from build123d import *

# Parameters (mm, degrees)
SKETCH1_R          = 1.3716
SKETCH1_R_2        = 1.905
SKETCH1_W          = 21.654448346
SKETCH1_H          = 40.81550601
EXTRUDE1_DEPTH     = 6.35
SKETCH2_R          = 2.032
EXTRUDE2_DEPTH     = 12.7
SKETCH3_R          = 1.349669532
CUT_EXTRUDE1_DEPTH = 72.389643478
SKETCH4_W          = 8.536869312
SKETCH4_H          = 4.372972384
CUT_EXTRUDE2_DEPTH = 72.389643478


with BuildPart() as part:
    # Sketch1 → Extrude1 (new, symmetric)
    with BuildSketch(Plane.XY):
        with BuildLine():
            Line((22.563049012, -49.803089557), (46.777222737, -43.035560041))
            ThreePointArc((46.777222737, -43.035560041), (49.511252826, -38.871621578), (45.757317366, -35.59728613))
            Line((45.757317366, -35.59728613), (24.862986263, -35.59728613))
            ThreePointArc((24.862986263, -35.59728613), (22.168909426, -34.481362966), (21.052986263, -31.78728613))
            Line((21.052986263, -31.78728613), (21.052986263, -18.898003738))
            ThreePointArc((21.052986263, -18.898003738), (22.168909426, -16.203926902), (24.862986263, -15.088003738))
            Line((24.862986263, -15.088003738), (31.554570289, -15.088003738))
            ThreePointArc((31.554570289, -15.088003738), (36.166042792, -10.476531235), (31.554570289, -5.865058732))
            Line((31.554570289, -5.865058732), (24.862986263, -5.865058732))
            ThreePointArc((24.862986263, -5.865058732), (22.168909426, -4.749135569), (21.052986263, -2.055058732))
            Line((21.052986263, -2.055058732), (21.052986263, 0.541184861))
            ThreePointArc((21.052986263, 0.541184861), (22.168909426, 3.235261698), (24.862986263, 4.351184861))
            Line((24.862986263, 4.351184861), (34.251425283, 4.351184861))
            Line((34.251425283, 4.351184861), (34.251425283, 11.107663069))
            Line((34.251425283, 11.107663069), (-34.251425283, 11.107663069))
            Line((-34.251425283, 11.107663069), (-34.251425283, 4.351184861))
            Line((-34.251425283, 4.351184861), (-24.862986263, 4.351184861))
            ThreePointArc((-24.862986263, 4.351184861), (-22.168909426, 3.235261698), (-21.052986263, 0.541184861))
            Line((-21.052986263, 0.541184861), (-21.052986263, -2.055058732))
            ThreePointArc((-21.052986263, -2.055058732), (-22.168909426, -4.749135569), (-24.862986263, -5.865058732))
            Line((-24.862986263, -5.865058732), (-31.554570289, -5.865058732))
            ThreePointArc((-31.554570289, -5.865058732), (-36.166042792, -10.476531235), (-31.554570289, -15.088003738))
            Line((-31.554570289, -15.088003738), (-24.862986263, -15.088003738))
            ThreePointArc((-24.862986263, -15.088003738), (-22.168909426, -16.203926902), (-21.052986263, -18.898003738))
            Line((-21.052986263, -18.898003738), (-21.052986263, -31.78728613))
            ThreePointArc((-21.052986263, -31.78728613), (-22.168909426, -34.481362966), (-24.862986263, -35.59728613))
            Line((-24.862986263, -35.59728613), (-45.757317366, -35.59728613))
            ThreePointArc((-45.757317366, -35.59728613), (-49.511252826, -38.871621578), (-46.777222737, -43.035560041))
            Line((-46.777222737, -43.035560041), (-22.563049012, -49.803089557))
            Line((-22.563049012, -49.803089557), (22.563049012, -49.803089557))
        make_face()
        with Locations((45.757317366, -39.38634569)):
            Circle(SKETCH1_R, mode=Mode.SUBTRACT)
        with Locations((31.554570289, -10.476531235)):
            Circle(SKETCH1_R_2, mode=Mode.SUBTRACT)
        with Locations(Location((-31.554570289, -10.476531235, 0), (0, 0, 180))):
            Circle(SKETCH1_R_2, mode=Mode.SUBTRACT)
        with Locations(Location((-45.757317366, -39.38634569, 0), (0, 0, 180))):
            Circle(SKETCH1_R, mode=Mode.SUBTRACT)
        with Locations((0.010545216, -19.616016269)):
            Rectangle(SKETCH1_W, SKETCH1_H, mode=Mode.SUBTRACT)
    extrude(amount=EXTRUDE1_DEPTH, both=True)

    # Sketch2 → Extrude2 (cut)
    with BuildSketch(Plane(origin=(0, 11.107663069, 0), x_dir=(1, 0, 0), z_dir=(0, 1, 0))):
        with Locations(Location((28.407237147, 0, 0), (0, 0, 180))):
            Circle(SKETCH2_R)
        with Locations(Location((-28.407237147, 0, 0), (0, 0, 270))):
            Circle(SKETCH2_R)
    extrude(amount=-EXTRUDE2_DEPTH, mode=Mode.SUBTRACT)

    # Sketch3 → Cut-Extrude1 (cut, through all)
    with BuildSketch(Plane.XY.offset(6.35)):
        with Locations((-15.402624173, -25.342644934)):
            Circle(SKETCH3_R)
        with Locations(Location((15.402624173, -25.342644934, 0), (0, 0, 180))):
            Circle(SKETCH3_R)
    extrude(amount=-CUT_EXTRUDE1_DEPTH, mode=Mode.SUBTRACT)

    # Sketch4 → Cut-Extrude2 (cut, through all)
    with BuildSketch(Plane.XY.offset(6.35)):
        with Locations((0.010545216, 0.791736736)):
            Rectangle(SKETCH4_W, SKETCH4_H)
    extrude(amount=-CUT_EXTRUDE2_DEPTH, mode=Mode.SUBTRACT)


solid = part.part
Input: part model. Units: mm. Frame: model coordinates. A direction names the side the tool comes from. Give positions to 0.01 mm unless a question says otherwise; leave off trailing zeros. Write each loop counter-clockwise with the first axis right and the second up, starting at its lowest first coordinate (ties: lowest second). Pieces come first, ordered by that corner, then holes.
Q1. First-contact query: P1, Ø1, axis at y = -8, z = -2, coming from the +X side; P2, Ø4, axis at x = 27.5, z = -1.5, coming from the -Y side; P3, Ø2.5, axis at x = 28.41, z = 0, coming from the -Y side; P4, Ø4, axis at y = -40.5, z = 2.5, coming from the -X side. Flat tips, straight axial feed; report the tip coordinate or a pass-through.
Q2. Pull-direction query (Z, two-part tool) for faces 1 (the face through (-12, -19, 6.35)), 2 (the face through (-26.7, 7.8, 1.1)), 3 (the face through (22.2, -4.78, 0.09)); classes: pulls with the +Z half, pulls with the -Z half, needs draft (parallel to the pull), parting line crosses it, or undercut.
Q3. Section C-C, the plane y = -34.5. Output: boundary loops of the cut face in (x, z), plus the area to 3 significant figures.
Q4. Material intervals for probe 1 along Y at (x, z) = (-6.5, -0.75); probe 2 along Z at (x, y) = (-28.5, 8); probe 3 along X at (y, z) = (-27.5, 3), sorted ascending.
Q5. Section D-D, the plane y = 6. Output: boundary loops of the cut face in (x, z).
Q6. Set-up query: faces 4 (the face through (22.139, -16.234, 0.089)), 5 (the face through (-22.14, -4.72, 0.09)), 6 (the face through (8, 0.792, 0)), 7 (the face through (0, 11.108, 0)). Return all of +Z, -Z, +X, -X, +Y, -Y with unobstructed straight access to the full face (end or side cutting, diameter ignored); none if empty.
Q7. Section A-A, the plane x = -7. Output: boundary loops of the cut face in (y, z), plus the area to 3 significant figures.
Q8. Section B-B, the plane z = 0. State how many separate pieces and enclosed holes the cut face has, plus the area to 3 significant figures.
Filled in:
1. P1: stops at x = 35.72
1. P2: stops at y = -48.98
1. P3: stops at y = -48.52
1. P4: stops at x = -49.55
2. face 1: pulls with the +Z half
2. face 2: undercut
2. face 3: needs draft
3. outline: (-22.19, -6.35) - (-10.82, -6.35) - (-10.82, 6.35) - (-22.19, 6.35) - close; (10.84, -6.35) - (22.19, -6.35) - (22.19, 6.35) - (10.84, 6.35) - close
3. area: 289 mm2
4. probe 1: y = -49.8 to -40.02, 0.79 to 11.11
4. probe 2: z = -6.35 to -2.03, 2.03 to 6.35
4. probe 3: x = -21.05 to -10.82, 10.84 to 21.05
5. outline: (-34.25, -6.35) - (34.25, -6.35) - (34.25, 6.35) - (-34.25, 6.35) - close; hole circle Ø4.06 at (-28.41, 0); hole circle Ø4.06 at (28.41, 0)
6. face 4: +Z, -Z, +X
6. face 5: +Z, -Z, -X
6. face 6: +Z, -Z
6. face 7: +Z, -Z, +X, -X, +Y
7. outline: (-49.8, -6.35) - (-40.02, -6.35) - (-40.02, 6.35) - (-49.8, 6.35) - close; (0.79, -6.35) - (11.11, -6.35) - (11.11, 6.35) - (0.79, 6.35) - close
7. area: 255 mm2
8. separate pieces: 3
8. enclosed holes: 7
8. area: 2,620 mm2
